Build history of the part. All positions in model axes, mm. Face numbers are marked on the shaded views. A direction names the side the tool comes from. Round coordinates to 2 decimals unless told otherwise and drop trailing zeros. Write each loop counter-clockwise with the first axis right and the second up, starting at its lowest first coordinate (ties: lowest second). Pieces come first, ordered by that corner, then holes. Notation, with made-up numbers: (10.25, 77) - (28.25, 77) arc R18 ccw to (28.25, 102) - close; hole circle Ø10 at (-16, 78). An arc over 180 degrees is marked (long way). Answer as a JSON object with one key per item and string values. Group by question number.
Item 1: Probe line 1 (Z direction, x = 27.15, y = 20.5); line 2 (X direction, y = 65, z = 0); line 3 (X direction, y = 46, z = 0). List the from-to ranges inside material, lowest first. Write a range as from..to.
Item 2: Two-plate mould, pull along X, no slides. Class the marked faces 1, 2 and 3: +X half, -X half, draft (parallel to the pull), parting line (faces both ways), or undercut.
Item 3: Flat gauge pins, fed straight in: pin 1 (3 mm diameter, centred on y = 1.5, z = -2.5, fed in from -X); pin 2 (18.5 mm diameter, centred on y = 27, z = 4.5, fed in from +X); pin 3 (3 mm diameter, centred on x = 27.15, z = -8.25, fed in from -Y). Where does each tip first touch, or does it go through?
Item 4: Which spindle directions (+Z, -Z, +X, -X, +Y, -Y) get a long thin tool onto all of the face, cutting with end or side? Do the marked faces 4, 5 and 6. Say none if no direction does.
Item 5: Slice it at A-A, the plane z = 0. Give the number of separate pieces and of enclosed holes in the cut face, then the cut area to 3 significant figures.
Item 6: Slice it at C-C, the plane x = -7. List the corners of the cut face in (y, z) (1 decimal), then the cut area to 3 significant figures.
Item 7: Slice it at D-D, the plane z = -17.5. List the corners of the cut face in (x, y), then the cut area to 3 significant figures.
Item 8: Slice it at B-B, the plane y = 91. List the corners of the cut face in (x, z).
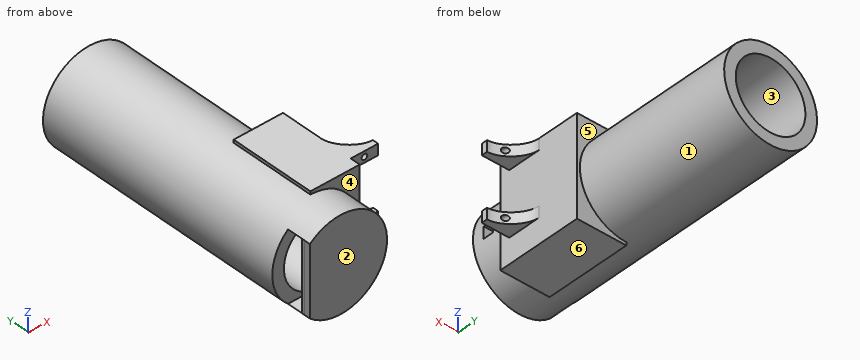
from build123d import *

# Parameters (mm, degrees)
SKETCH1_R                = 20
BOSS_EXTRUDE1_DEPTH      = 120.5
BOSS_EXTRUDE2_START      = 14.5
BOSS_EXTRUDE2_DEPTH      = 36.8
SKETCH7_W                = 4.7
SKETCH7_H                = 2.5
BOSS_EXTRUDE3_DEPTH      = 11.8
SKETCH2_R                = 15
CUT_EXTRUDE2_DEPTH       = 115.5
CUT_EXTRUDE3_REACH       = 135.373
CUT_EXTRUDE3_END_RADIUS  = 15
SKETCH12_W               = 30
SKETCH12_H               = 5.5
CUT_EXTRUDE5_DEPTH       = 5
FILLET3_SIZE             = 2.5
M2_CLEARANCE_HOLE3_D     = 2.4
M2_CLEARANCE_HOLE3_DEPTH = 2.5
M2_CLEARANCE_HOLE3_TIP   = 0.721032743
FILLET4_SIZE             = 11.8
CUT_EXTRUDE6_REACH       = 130.74
CUT_EXTRUDE6_END_RADIUS  = 15


with BuildPart() as part:
    # Sketch1 → Boss-Extrude1 (new body)
    with BuildSketch(Plane(origin=(0, 0, 0), x_dir=(1, 0, 0), z_dir=(0, 1, 0))):
        with Locations(Location((0, 0, 0), (0, 0, 270))):
            Circle(SKETCH1_R)
    extrude(amount=BOSS_EXTRUDE1_DEPTH)

    # Sketch6 → Boss-Extrude2 (add)
    with BuildSketch(Plane(origin=(0, 0, 0), x_dir=(1, 0, 0), z_dir=(0, 1, 0)).offset(BOSS_EXTRUDE2_START)):
        Polygon((21.25, 21.3), (21.25, 0), (21.25, -21.3), (0, -21.3), (0, 0), (0, 21.3), align=None)
    extrude(amount=BOSS_EXTRUDE2_DEPTH)

    # Sketch7 → Boss-Extrude3 (add)
    with BuildSketch(Plane(origin=(21.25, 0, 0), x_dir=(0, 0, -1), z_dir=(1, 0, 0))):
        with Locations((8.25, 20.05)):
            Rectangle(SKETCH7_W, SKETCH7_H)
        with Locations((-18.95, 20.05)):
            Rectangle(SKETCH7_W, SKETCH7_H)
    extrude(amount=BOSS_EXTRUDE3_DEPTH)

    # Sketch2 → Cut-Extrude2 (cut)
    with BuildSketch(Plane(origin=(0, 120.5, 0), x_dir=(1, 0, 0), z_dir=(0, 1, 0))):
        with Locations(Location((0, 0, 0), (0, 0, 270))):
            Circle(SKETCH2_R)
    extrude(amount=-CUT_EXTRUDE2_DEPTH, mode=Mode.SUBTRACT)

    # Cut-Extrude3: up to this cylinder (the profile starts outside it)
    cut_extrude3_end = Plane(origin=(0, 7.75, 0), z_dir=(0, 1, 0)) * Cylinder(CUT_EXTRUDE3_END_RADIUS, 301.746, mode=Mode.PRIVATE)
    # Sketch12 → Cut-Extrude3 (cut, up to the surface)
    with BuildSketch(Plane.ZY.offset(20), mode=Mode.PRIVATE) as cut_extrude3_sk1:
        with Locations((0, 7.75)):
            Rectangle(SKETCH12_W, SKETCH12_H)
    cut_extrude3_tool1 = extrude(cut_extrude3_sk1.sketch, amount=-CUT_EXTRUDE3_REACH, mode=Mode.PRIVATE) - cut_extrude3_end
    add(cut_extrude3_tool1.solids().sort_by_distance((-20, 7.75, 0))[0], mode=Mode.SUBTRACT)

    # Sketch13 → Cut-Extrude5 (cut)
    with BuildSketch(Plane.XZ):
        with BuildLine():
            Line((-13.228756555, 15), (-13.228756555, -15))
            ThreePointArc((-13.228756555, -15), (-20, 0), (-13.228756555, 15))
        make_face()
    extrude(amount=-CUT_EXTRUDE5_DEPTH, mode=Mode.SUBTRACT)

    # Fillet3
    # a fillet whose section is not a circle: 2.5 mm, written as the material it takes off along each edge
    with BuildSketch(Plane(origin=(-13.228756555, 5, 15), x_dir=(0, -1, 0), z_dir=(0, 0, -1))) as fillet3_piece_1:
        with BuildLine():
            Bezier((FILLET3_SIZE, 0), (0, 0), (0, -FILLET3_SIZE), weights=[1, 1.222222222, 1])
            Line((0, -FILLET3_SIZE), (0, 0))
            Line((0, 0), (FILLET3_SIZE, 0))
        make_face()
    extrude(amount=30, mode=Mode.SUBTRACT)

    # M2 Clearance Hole3
    with Locations(Plane(origin=(0, 18.8, 0), x_dir=(-1, 0, 0), z_dir=(0, -1, 0))):
        with Locations((-27.15, 8.25), (-27.15, -18.95)):
            Hole(M2_CLEARANCE_HOLE3_D / 2, depth=M2_CLEARANCE_HOLE3_DEPTH)
            with Locations((0, 0, -(M2_CLEARANCE_HOLE3_DEPTH + M2_CLEARANCE_HOLE3_TIP / 2))):  # 118° drill point
                Cone(0, M2_CLEARANCE_HOLE3_D / 2, M2_CLEARANCE_HOLE3_TIP, mode=Mode.SUBTRACT)

    # Fillet4
    # a fillet whose section is not a circle: 11.8 mm, written as the material it adds along each edge
    with BuildSketch(Plane(origin=(21.25, 21.3, 21.3), x_dir=(1, 0, 0), z_dir=(0, 0, -1))) as fillet4_piece_1_section:
        with BuildLine():
            Bezier((FILLET4_SIZE, 0), (0, 0), (0, -FILLET4_SIZE), weights=[1, 0.538461538, 1])
            Line((0, -FILLET4_SIZE), (0, 0))
            Line((0, 0), (FILLET4_SIZE, 0))
        make_face()
    fillet4_piece_1 = extrude(amount=4.7, mode=Mode.PRIVATE)
    fillet4_piece_1 = fillet4_piece_1 - Plane(origin=(27.15, 21.3, 18.95), x_dir=(1, 0, 0), z_dir=(0, 1, 0)) * Cylinder(1.2, 57, mode=Mode.PRIVATE)
    add(fillet4_piece_1)
    with BuildSketch(Plane(origin=(21.25, 21.3, 21.3), x_dir=(1, 0, 0), z_dir=(0, 0, -1))) as fillet4_piece_2_section:
        with BuildLine():
            Bezier((FILLET4_SIZE, 0), (0, 0), (0, -FILLET4_SIZE), weights=[1, 0.538461538, 1])
            Line((0, -FILLET4_SIZE), (0, 0))
            Line((0, 0), (FILLET4_SIZE, 0))
        make_face()
    fillet4_piece_2 = extrude(amount=34.2, mode=Mode.PRIVATE)
    fillet4_piece_2 = split(fillet4_piece_2, bisect_by=Plane(origin=(21.25, 21.3, -5.9), z_dir=(0, 0, -1)), keep=Keep.TOP, mode=Mode.PRIVATE)
    fillet4_piece_2 = split(fillet4_piece_2, bisect_by=Plane(origin=(21.25, 21.3, -10.6), z_dir=(0, 0, 1)), keep=Keep.TOP, mode=Mode.PRIVATE)
    fillet4_piece_2 = fillet4_piece_2 - Plane(origin=(27.15, 21.3, -8.25), x_dir=(1, 0, 0), z_dir=(0, 1, 0)) * Cylinder(1.2, 116, mode=Mode.PRIVATE)
    add(fillet4_piece_2)
    with BuildSketch(Plane(origin=(21.25, 21.3, -10.6), x_dir=(0, 1, 0), z_dir=(0, 0, 1))) as fillet4_piece_3_section:
        with BuildLine():
            Bezier((FILLET4_SIZE, 0), (0, 0), (0, -FILLET4_SIZE), weights=[1, 0.538461538, 1])
            Line((0, -FILLET4_SIZE), (0, 0))
            Line((0, 0), (FILLET4_SIZE, 0))
        make_face()
    fillet4_piece_3 = extrude(amount=4.7, mode=Mode.PRIVATE)
    fillet4_piece_3 = fillet4_piece_3 - Plane(origin=(27.15, 21.3, -8.25), x_dir=(1, 0, 0), z_dir=(0, 1, 0)) * Cylinder(1.2, 57, mode=Mode.PRIVATE)
    add(fillet4_piece_3)
    with BuildSketch(Plane(origin=(21.25, 21.3, -10.6), x_dir=(0, 1, 0), z_dir=(0, 0, 1))) as fillet4_piece_4_section:
        with BuildLine():
            Bezier((FILLET4_SIZE, 0), (0, 0), (0, -FILLET4_SIZE), weights=[1, 0.538461538, 1])
            Line((0, -FILLET4_SIZE), (0, 0))
            Line((0, 0), (FILLET4_SIZE, 0))
        make_face()
    fillet4_piece_4 = extrude(amount=34.2, mode=Mode.PRIVATE)
    fillet4_piece_4 = split(fillet4_piece_4, bisect_by=Plane(origin=(21.25, 21.3, 21.3), z_dir=(0, 0, -1)), keep=Keep.TOP, mode=Mode.PRIVATE)
    fillet4_piece_4 = split(fillet4_piece_4, bisect_by=Plane(origin=(21.25, 21.3, 16.6), z_dir=(0, 0, 1)), keep=Keep.TOP, mode=Mode.PRIVATE)
    fillet4_piece_4 = fillet4_piece_4 - Plane(origin=(27.15, 21.3, 18.95), x_dir=(1, 0, 0), z_dir=(0, 1, 0)) * Cylinder(1.2, 116, mode=Mode.PRIVATE)
    add(fillet4_piece_4)

    # Cut-Extrude6: up to this cylinder (the profile starts outside it)
    cut_extrude6_end = Plane(origin=(0, 7.25, 0), z_dir=(0, 1, 0)) * Cylinder(CUT_EXTRUDE6_END_RADIUS, 292.48, mode=Mode.PRIVATE)
    # Sketch21 → Cut-Extrude6 (cut, up to the surface)
    with BuildSketch(Plane(origin=(20, 0, 0), x_dir=(0, 0, -1), z_dir=(1, 0, 0)), mode=Mode.PRIVATE) as cut_extrude6_sk1:
        Polygon((0, 5), (-2.5, 5), (-2.5, 9.5), (2.5, 9.5), (2.5, 5), align=None)
    cut_extrude6_tool1 = extrude(cut_extrude6_sk1.sketch, amount=-CUT_EXTRUDE6_REACH, mode=Mode.PRIVATE) - cut_extrude6_end
    add(cut_extrude6_tool1.solids().sort_by_distance((20, 7.25, 0))[0], mode=Mode.SUBTRACT)


solid = part.part
Geometry says:
{
 "1": {"line 1": "z = -10.6..-9.45, -7.05..-5.9, 16.6..17.75, 20.15..21.3", "line 2": "x = -20..-15, 15..20", "line 3": "x = -20..-15, 15..21.25"},
 "2": {"face 1": "parting line", "face 2": "draft", "face 3": "undercut"},
 "3": {"pin 1": "stops at x = -13.23", "pin 2": "stops at x = 21.25", "pin 3": "stops at y = 18.8"},
 "4": {"face 4": "+X, -Y", "face 5": "+X, +Y", "face 6": "-Z, +X, -X, +Y, -Y"},
 "5": {"separate pieces": "3", "enclosed holes": "0", "area": "1,320 mm^2"},
 "6": {"outline": "(0, -18.7) - (120.5, -18.7) - (120.5, -13.3) - (10.5, -13.3) - (10.5, -15) - (5, -15) - (5, 15) - (10.5, 15) - (10.5, 13.3) - (120.5, 13.3) - (120.5, 18.7) - (0, 18.7) - close", "area": "1,430 mm^2"},
 "7": {"outline": "(-9.68, 0) - (9.68, 0) - (9.68, 14.5) - (21.25, 14.5) - (21.25, 51.3) - (9.68, 51.3) - (9.68, 120.5) - (-9.68, 120.5) - close", "area": "2,760 mm^2"},
 "8": {"outline": "circle Ø40 at (0, 0); hole circle Ø30 at (0, 0)"}
}
